Autodesk Inventor part; units mm, degrees
ref_plane "Start Plane" through (0, 0, 0) normal (0, 0, 1) x (1, 0, 0)
ref_plane "End Plane" through (0, 0, 551.5) normal (0, 0, 1) x (1, 0, 0)
ref_plane "Work Plane5" through (0, 15, 551.5) normal (0, -0.7071, 0.7071) x (1, 0, 0)
ref_plane "Start Plane" through (0, 0, 0) normal (0, 0, 1) x (1, 0, 0)
ref_plane "End Plane" through (0, 0, 551.5) normal (0, 0, 1) x (1, 0, 0)
sketch "Sketch" plane through (0, 0, 0) normal (0, 0, 1) x (1, 0, 0)
  line L0 (-15, -9) -> (-15, 9)
  line L1 (-9, 15) -> (9, 15)
  line L2 (15, 9) -> (15, -9)
  line L3 (9, -15) -> (-9, -15)
  arc A0 (-15, -9) -> (-9, -15) centre (-9, -9) ccw
  arc A1 (-9, 15) -> (-15, 9) centre (-9, 9) ccw
  arc A2 (15, 9) -> (9, 15) centre (9, 9) ccw
  arc A3 (9, -15) -> (15, -9) centre (9, -9) ccw
  arc A4 (-9, 12) -> (-12, 9) centre (-9, 9) ccw
  line L4 (-9, 12) -> (9, 12)
  arc A5 (12, 9) -> (9, 12) centre (9, 9) ccw
  line L5 (12, 9) -> (12, -9)
  arc A6 (9, -12) -> (12, -9) centre (9, -9) ccw
  line L6 (9, -12) -> (-9, -12)
  arc A7 (-12, -9) -> (-9, -12) centre (-9, -9) ccw
  line L7 (-12, -9) -> (-12, 9)
  line L8 (0, 22.7397) -> (0, -22.7397) construction
  line L9 (-22.7397, 0) -> (22.7397, 0) construction
  dimension "d7" = 6
  dimension "d10" = 30
  dimension "d11" = 30
  dimension "d12" = 3
  dimension "d15" = 15
  dimension "d16" = 15
extrude "Body" add sketch "Sketch" along normal up to surface (551.5 mm away) from surface at 0
sketch "Sketch3" plane through (0, 0, 0) normal (0, 0, 1) x (1, 0, 0)
  line L0 (0, 0) -> (10, 0)
ref_plane "Work Plane3" through (0, 0, 0) normal (0, -1, 0) x (1, 0, 0)
ref_plane "Work Plane5" through (0, 15, 551.5) normal (0, -0.7071, 0.7071) x (1, 0, 0)
split "Split2" plane through (0, 15, 551.5) removes the side toward (0, -0.7071, 0.7071)
sketch "Sketch4" plane through (0, 0, 0) normal (0, -1, 0) x (1, 0, 0)
  line L0 (-2, 0) -> (12, 0)
  line L1 (-2, 551.5) -> (12, 551.5)
  dimension "d18" = 551.5
equation "\"d7\" = G_IR"
equation "\"d10\" = G_H"
equation "\"d11\" = G_W"
equation "\"d12\" = G_T"
equation "\"d15\" = 0.5 * d10"
equation "\"d16\" = 0.5 * d11"
equation "\"d3\" = G_L"
equation "\"G_W\" = 30"
equation "\"G_H\" = 30"
equation "\"G_T\" = 3"
equation "\"G_IR\" = 6"
equation "\"G_L\" = d18"
equation "\"G_OFFSET_START\" = 0"
equation "\"G_OFFSET_END\" = 15"
equation "\"d14\" = G_OFFSET_END + B_L"
equation "\"B_L\" = 536.5"
properties part number "DIN EN 10219-2 - 30 x 30 x 3  - 551.5" material "Steel, Mild"
Design review of the part built by this model. Coordinates are the model's own, in mm. A direction names the side the tool comes from. Round coordinates to 2 decimals unless told otherwise and drop trailing zeros. Write each loop counter-clockwise with the first axis right and the second up, starting at its lowest first coordinate (ties: lowest second). Pieces come first, ordered by that corner, then holes. Notation, with made-up numbers: M 83.25,-4 L 125.25,-4 A30 ccw 125.25,32 Z; hole C 68,-20 d3. An arc over 180 degrees is marked long. One line per item, written item: value. Start each with the question number.
1. Take a section at B-B on z = 112.5. State the section outline as (x, y) points.
2. To check wall thickness, follow probe 1 along Y at (x, z) = (7.75, 439.5); probe 2 along Z at (x, y) = (-2.25, 13.5). State the ranges of each line that lie inside material, in increasing order. Write a range as from..to.
3. Take a section at A-A on y = -3.5. State the section outline as (x, z) points, then the cut area to 3 significant figures.
4. Draft analysis for pull direction X (two halves, no side actions). For faces 3 (the face through (12, 0, 269)), 4 (the face through (0, 15, 272)), 5 (the face through (-15, 0, 269)), state which applies: pulls with the +X half, pulls with the -X half, needs draft (parallel to the pull), parting line crosses it, or undercut.
5. For faces 1 (the face through (15, 0, 269)), 2 (the face through (0, -12, 259)), list the 3-axis set-ups (+Z, -Z, +X, -X, +Y, -Y) from which the entire face can be reached by the end or side of a thin tool; tool diameter is ignored.
Computed:
1. outline: M -15,-9 A6 ccw -9,-15 L 9,-15 A6 ccw 15,-9 L 15,9 A6 ccw 9,15 L -9,15 A6 ccw -15,9 Z; hole M -12,-9 A3 ccw -9,-12 L 9,-12 A3 ccw 12,-9 L 12,9 A3 ccw 9,12 L -9,12 A3 ccw -12,9 Z
2. probe 1: y = -15..-12, 12..15
2. probe 2: z = 0..550
3. outline: M -15,0 L -12,0 L -12,533 L -15,533 Z; M 12,0 L 15,0 L 15,533 L 12,533 Z
3. area: 3,200 mm²
4. face 3: undercut
4. face 4: needs draft
4. face 5: pulls with the -X half
5. face 1: +Z, -Z, +X, +Y, -Y
5. face 2: +Z, -Z
